Work out the finished part from the listing and answer in its coordinate system (mm). Round coordinates to 2 decimals unless told otherwise and drop trailing zeros. Order: outer loops, then holes, each group sorted by start corner. A loop starts at its lowest first (then second) coordinate and runs counter-clockwise, first axis right, second up.
from build123d import *

# Parameters (mm, degrees)
SKETCH1_W               = 457.2
SKETCH1_H               = 330.2
BOSS_EXTRUDE1_DEPTH     = 12.7
F_3_8_CLEARANCE_HOLE1_D = 10.0838


with BuildPart() as part:
    # Sketch1 → Boss-Extrude1 (new body)
    with BuildSketch(Plane(origin=(0, 0, 0), x_dir=(1, 0, 0), z_dir=(0, 1, 0))):
        Rectangle(SKETCH1_W, SKETCH1_H)
    extrude(amount=BOSS_EXTRUDE1_DEPTH)

    # 3/8 Clearance Hole1 (through all)
    with Locations(Plane(origin=(0, 12.7, -165.1), x_dir=(1, 0, 0), z_dir=(0, 1, 0))):
        with Locations((-114.300000003, -88.9), (-114.300000003, -190.5), (-114.300000003, -292.1)):
            Hole(F_3_8_CLEARANCE_HOLE1_D / 2)


solid = part.part
Item 1: Find the intervals of material crossed by line 1 along Z through (x, y) = (-114.3, 8), in increasing order.
Item 2: Given pin 1 (4 mm diameter, centred on x = -62, z = 66, fed in from -Y); pin 2 (8 mm diameter, centred on x = -114.3, z = -76.2, fed in from +Y), each flat-ended and moving along its own axis, determine where each tip first touches the part or whether it passes through.
Item 3: Find section A-A (x = -114.3). Write down the section's boundary in (y, z), plus the area to 3 significant figures.
Item 4: Find section B-B (z = 127). Write down the section's boundary in (x, y).
Item 5: For a pull along Z with two mould halves and no side action, classify faces 1 (the face through (-119.11, 6.26, 125.49)), 2 (the face through (228.6, 6, 2)), 3 (the face through (-3, 6, 165.1)), 4 (the face through (-118.96, 6.26, -74.27)) as released by +Z, released by -Z, zero draft, split by the parting line, or undercut.
Model answer:
1. line 1: z = -165.1 to -81.24, -71.16 to 20.36, 30.44 to 121.96, 132.04 to 165.1
2. pin 1: stops at y = 0
2. pin 2: passes through
3. outline: (0, -165.1) - (12.7, -165.1) - (12.7, -81.24) - (0, -81.24) - close; (0, -71.16) - (12.7, -71.16) - (12.7, 20.36) - (0, 20.36) - close; (0, 30.44) - (12.7, 30.44) - (12.7, 121.96) - (0, 121.96) - close; (0, 132.04) - (12.7, 132.04) - (12.7, 165.1) - (0, 165.1) - close
3. area: 3,810 mm2
4. outline: (-228.6, 0) - (-119.34, 0) - (-119.34, 12.7) - (-228.6, 12.7) - close; (-109.26, 0) - (228.6, 0) - (228.6, 12.7) - (-109.26, 12.7) - close
5. face 1: undercut
5. face 2: zero draft
5. face 3: released by +Z
5. face 4: undercut
